Input: part model. Units: mm. Frame: model coordinates. A direction names the side the tool comes from. Coordinates: 2 decimals unless noted, no trailing zeros. Use a Markdown table: item, result. Add a question column.
Q1. Material intervals for probe 1 along Z at (x, y) = (0.5, 14); probe 2 along X at (y, z) = (-1.5, -4.75); probe 3 along X at (y, z) = (2, -4.5), sorted ascending. Write a range as from..to.
Q2. Mould query, pull axis Y, two halves, no side actions, for faces 3 (the face through (0, -11, -0.1)), 4 (the face through (-11, 0, -0.1)), 5 (the face through (-8, 8, -5)), 6 (the face through (-3.794, 17.084, -3.986)). Classes: released by +Y, released by -Y, zero draft, split by the parting line, or undercut.
Q3. Pin query (flat end, axial travel): P1, Ø2, axis at y = 4, z = -1, coming from the -X side; P2, Ø12, axis at x = 4.5, y = 8.5, coming from the +Z side; P3, Ø1, axis at y = 4, z = -3, coming from the +X side; P4, Ø2.5, axis at x = 0, y = -10.98, coming from the -Z side. Return the tip coordinate at first contact, or that it passes through.
Q4. Set-up query: faces 1 (the face through (6, 6, 0)), 2 (the face through (0, 11, -0.1)). Return all of +Z, -Z, +X, -X, +Y, -Y with unobstructed straight access to the full face (end or side cutting, diameter ignored); none if empty.
from build123d import *

# Parameters (mm, degrees)
FILETE1_R             = 3
ESBO_O2_R             = 2.209069454
CORTE_EXTRUS_O1_DEPTH = 0.1
PADR_OCIRCULAR1_COUNT = 4
FILETE2_R             = 1


with BuildPart() as part:
    # Esboço1 → Revolução1 (revolve)
    with BuildSketch(Plane(origin=(0, 0, 0), x_dir=(0, 0, -1), z_dir=(1, 0, 0)), mode=Mode.PRIVATE) as revolu_o1_sk:
        Polygon((6.5, 4.25), (6.5, 8.25), (5, 9.5), (5, 17.5), (0, 17.5), (0, 8), (1, 8), (5.5, 4.25), align=None)
    revolve(revolu_o1_sk.sketch.rotate(Axis((0, 0, 0), (0, 0, -1)), 90), axis=Axis((0, 0, 0), (0, 0, -1)))

    # Filete1
    filete1_edges = [part.edges().sort_by_distance(p)[0] for p in [
        (-17.5, 0, 0),
    ]]
    fillet(filete1_edges, radius=FILETE1_R)

    # Esboço2 → Corte-extrusão1 (cut)
    with BuildSketch(Plane.XY):
        with Locations((0, 10.983322756)):
            Circle(ESBO_O2_R)
    corte_extrus_o1 = extrude(amount=-CORTE_EXTRUS_O1_DEPTH, mode=Mode.SUBTRACT)

    # PadrãoCircular1: Corte-extrusão1 ×4 about axis
    padr_ocircular1_axis = Axis((0, 0, 0), (0, 0, 1))
    for i in range(1, PADR_OCIRCULAR1_COUNT):
        add(corte_extrus_o1.rotate(padr_ocircular1_axis, i * 360 / PADR_OCIRCULAR1_COUNT), mode=Mode.SUBTRACT)

    # Filete2
    filete2_edges = [part.edges().sort_by_distance(p)[0] for p in [
        (-9.5, 0, -5),
        (-8.25, 0, -6.5),
    ]]
    fillet(filete2_edges, radius=FILETE2_R)


solid = part.part
Values follow:
| question | item | result |
|---|---|---|
| 1 | probe 1 | -5..0 |
| 1 | probe 2 | -17.44..-4.64, 4.64..17.44 |
| 1 | probe 3 | -17.39..-4.67, 4.67..17.39 |
| 2 | face 3 | undercut |
| 2 | face 4 | undercut |
| 2 | face 5 | zero draft |
| 2 | face 6 | split by the parting line |
| 3 | P1 | x = -16.92 |
| 3 | P2 | z = 0 |
| 3 | P3 | x = 17.15 |
| 3 | P4 | z = -5.03 |
| 4 | face 1 | +Z, +X, -X, +Y, -Y |
| 4 | face 2 | +Z |
